Could you check a few things on this model? Use its own coordinates, in mm. Face numbers are marked on the shaded views. A direction names the side the tool comes from. Coordinates: 2 decimals unless noted, no trailing zeros. Order: outer loops, then holes, each group sorted by start corner. A loop starts at its lowest first (then second) coordinate and runs counter-clockwise, first axis right, second up. Notation, with made-up numbers: (44, 77) - (81, 77) arc R20 cw to (81, 112) - close; hole circle Ø11 at (69, 89). An arc over 180 degrees is marked (long way). Answer as CSV lines item,"result". Start each with the question number.
1. I want a section at C-C, the plane z = 17.75. List the corners of the cut face in (x, y) for me.
2. For pin 1 (1.5 mm diameter, centred on y = 19, z = 19, fed in from -X); pin 2 (5 mm diameter, centred on x = -9.5, z = 3.5, fed in from +Y); pin 3 (2.5 mm diameter, centred on y = 18.5, z = 11, fed in from +X), each with a flat end and sliding along its axis, tell me the tip position at first contact or that it passes through.
3. I want a section at B-B, the plane y = 13.25. List the corners of the cut face in (x, z) for me.
4. Thinking about a two-plate mould opening in X: for the marked faces 4, 5 and 6, which applies, released by +X, released by -X, zero draft, split by the parting line, or undercut?
5. For the marked faces 1, 2 and 3, which set-ups out of +Z, -Z, +X, -X, +Y, -Y let a thin tool reach every point of the face, with its end or its side?
6. I want a section at D-D, the plane x = 12.5. List the corners of the cut face in (y, z) for me.
7. I want a section at A-A, the plane x = 24.5. List the corners of the cut face in (y, z) for me.
8. I need wall thicknesses on probe 1 along X at (y, z) = (3.1, 11); probe 2 along X at (y, z) = (22.55, 9); probe 3 along Z at (x, y) = (8, 22). Which ranges of each line are inside material? Lowest first, please.
Autodesk Fusion 360 part; units mm, degrees
sketch "Skizze1" plane through (0, 0, 0) normal (0, 0, 1) x (1, 0, 0)
  line L0 (0, 24) -> (16, 24)
  line L1 (16, 0) -> (0, 0)
  line L2 (2, 22) -> (14, 22)
  line L3 (0, 24) -> (-1, 24)
  line L4 (-1, 24) -> (-1, 0)
  line L5 (-1, 0) -> (0, 0)
  line L6 (16, 24) -> (17, 24)
  line L7 (17, 24) -> (17, 0)
  line L8 (17, 0) -> (16, 0)
  line L9 (2, 22) -> (1, 22)
  line L10 (1, 22) -> (1, 20)
  line L11 (1, 20) -> (2, 20)
  line L12 (15, 20) -> (15, 22)
  line L13 (15, 22) -> (14, 22)
  line L14 (15, 20) -> (2, 20)
  line L15 (2, 20) -> (2, 0)
  line L16 (14, 20) -> (14, 0)
extrude "Extrusion1" add sketch "Skizze1" along normal blind 2
sketch "Skizze2" plane through (0, 0, 2) normal (0, 0, 1) x (-1, 0, 0)
  line L0 (-17, -24) -> (1, -24)
  line L1 (1, -24) -> (1, 0)
  line L2 (1, 0) -> (-17, 0)
  line L3 (-17, 0) -> (-17, -24)
  line L4 (-2, 0) -> (-2, -20)
  line L5 (-2, -20) -> (-1, -20)
  line L6 (-1, -20) -> (-1, -22)
  line L7 (-1, -22) -> (-15, -22)
  line L8 (-15, -22) -> (-15, -20)
  line L9 (-15, -20) -> (-14, -20)
  line L10 (-14, -20) -> (-14, 0)
  line L11 (-2, -20) -> (-14, -20)
extrude "Extrusion2" add sketch "Skizze2" along normal blind 1 contours L0 L1 L2 L3 L4 L5 L6 L7 L8 L9 L10 | L2 L4 L10 L11
sketch "Skizze3" plane through (0, 0, 3) normal (0, 0, 1) x (-1, 0, 0)
  line L0 (-15, -20) -> (-1, -20)
  line L1 (-1, -20) -> (-1, -22)
  line L2 (-1, -22) -> (-15, -22)
  line L3 (-15, -22) -> (-15, -20)
  line L4 (-17, 0) -> (-17, -24)
  line L5 (-17, -24) -> (1, -24)
  line L6 (1, -24) -> (1, 0)
  line L7 (1, 0) -> (-17, 0)
  line L8 (-2, -20) -> (-2, 0)
  line L9 (-14, -20) -> (-14, 0)
extrude "Extrusion3" add sketch "Skizze3" along normal blind 19 contours L0 L1 L2 L3 L4 L5 L6 L7 L8 L9
sketch "Skizze4" plane through (0, 0, 22) normal (0, 0, 1) x (-1, 0, 0)
  line L0 (-2, -20) -> (-1, -20)
  line L1 (-1, -20) -> (-1, -22)
  line L2 (-1, -22) -> (-15, -22)
  line L3 (-15, -22) -> (-15, -20)
  line L4 (-15, -20) -> (-14, -20)
  line L5 (-14, -20) -> (-14, 0)
  line L6 (-14, 0) -> (-17, 0)
  line L7 (-17, 0) -> (-17, -24)
  line L8 (-17, -24) -> (1, -24)
  line L9 (1, -24) -> (1, 0)
  line L10 (1, 0) -> (-2, 0)
  line L11 (-2, 0) -> (-2, -20)
  line L12 (-2, -22) -> (-2, -24)
  line L13 (-14, -22) -> (-14, -24)
extrude "Extrusion4" cut sketch "Skizze4" against normal blind 19 contours L2 L8 L12 L13
sketch "Skizze5" plane through (0, 0, 3) normal (0, 0, 1) x (-1, 0, 0)
  line L0 (-14, 0) -> (-14, -20)
  line L1 (-14, -20) -> (-2, -20)
  line L2 (-2, -20) -> (-2, 0)
  line L3 (-2, 0) -> (-14, 0)
sketch "Skizze6" plane through (0, 0, 3) normal (0, 0, 1) x (1, 0, 0)
sketch "Skizze7" plane through (0, 0, 0) normal (0, 0, 1) x (1, 0, 0)
  line L0 (-1, 0) -> (-16, 0)
  line L1 (-16, 0) -> (-16, 5)
  line L2 (-16, 5) -> (-1, 5)
  line L3 (-1, 5) -> (-1, 0)
  line L4 (17, 0) -> (17, 5)
  line L5 (17, 5) -> (32, 5)
  line L6 (32, 5) -> (32, 0)
  line L7 (32, 0) -> (17, 0)
extrude "Extrusion5" add sketch "Skizze7" along normal blind 22
hole "Bohrung1" at (24.5, 5, 11) direction (0, -1, 0) diameter 2.5 depth 5 tip angle 180 countersink diameter 4.5 countersink angle 90
hole "Bohrung2" at (-8.5, 5, 11) direction (0, -1, 0) diameter 2.5 depth 5 tip angle 180 countersink diameter 4.5 countersink angle 90
extrude "Extrusion6" cut 1 faces at (14.6667, 20, 9) along direction (0, -1, 0) blind 1
extrude "Extrusion7" add 1 faces at (1.3333, 22, 9) along direction (0, -1, 0) blind 1
sketch "Skizze8" plane through (0, 0, 3) normal (0, 0, 1) x (-1, 0, 0)
  line L0 (-14, -21) -> (-14, -24)
  line L1 (-14, -24) -> (-2, -24)
  line L2 (-2, -24) -> (-2, -21)
  line L3 (-2, -21) -> (-14, -21)
  line L4 (-2, -23) -> (-14, -23)
  line L5 (-14, -23) -> (-14, -24)
  line L6 (-14, -24) -> (-2, -24)
  line L7 (-2, -24) -> (-2, -23)
  line L8 (-2, -23) -> (-14, -23)
  line L9 (-14, -23) -> (-14, -24)
extrude "Extrusion8" add sketch "Skizze8" along normal blind 19 contours L0 L1 L2 L4 L5 L6 L7 L8 L9
sketch "Skizze9" plane through (0, 24, 0) normal (0, 1, 0) x (-1, 0, 0)
  line L0 (1, 22) -> (-17, 22)
  line L1 (-17, 22) -> (-17, 0)
  line L2 (-17, 0) -> (1, 0)
  line L3 (1, 0) -> (1, 22)
  line L4 (-8, 0) -> (-8, 9)
hole "Bohrung3" at (8, 24, 9) direction (0, -1, 0) diameter 8 depth 9 tip angle 180
extrude "Extrusion9" cut 1 faces at (14.6667, 19, 9) along direction (0, -1, 0) blind 1.5
extrude "Extrusion10" add 1 faces at (1.3333, 21, 9) along direction (0, -1, 0) blind 1.4
extrude "Extrusion11" add 1 faces at (8, 23, 19) along direction (0, -1, 0) blind 1.2
extrude "Extrusion12" cut 1 faces at (8, 24, 19) along direction (0, -1, 0) blind 1.2
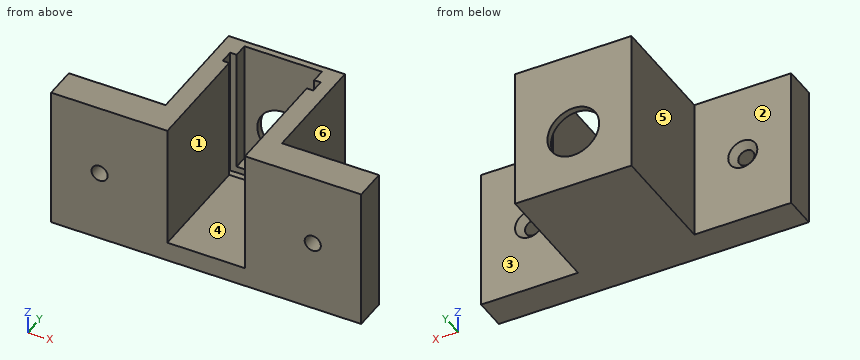
Solved:
1,outline,"(-16, 0) - (2, 0) - (2, 17.5) - (1, 17.5) - (1, 19.6) - (2, 19.6) - (2, 21.8) - (14, 21.8) - (14, 19.6) - (15, 19.6) - (15, 17.5) - (14, 17.5) - (14, 0) - (32, 0) - (32, 5) - (17, 5) - (17, 22.8) - (-1, 22.8) - (-1, 5) - (-16, 5) - close"
2,pin 1,"stops at x = -1"
2,pin 2,"stops at y = 5"
2,pin 3,"stops at x = 17"
3,outline,"(-1, 0) - (17, 0) - (17, 22) - (14, 22) - (14, 3) - (2, 3) - (2, 22) - (-1, 22) - close"
4,face 4,"undercut"
4,face 5,"released by -X"
4,face 6,"released by +X"
5,face 1,"+Z, -Y"
5,face 2,"+Z, -Z, -X, +Y"
5,face 3,"+Z, -Z, +X, +Y"
6,outline,"(0, 0) - (22.8, 0) - (22.8, 22) - (21.8, 22) - (21.8, 3) - (19.6, 3) - (19.6, 2) - (17.5, 2) - (17.5, 3) - (0, 3) - close"
7,outline,"(0, 0) - (5, 0) - (5, 8.75) - (4, 9.75) - (0, 9.75) - close; (0, 12.25) - (4, 12.25) - (5, 13.25) - (5, 22) - (0, 22) - close"
8,probe 1,"x = -16 to -9.75, -7.25 to 2, 14 to 23.25, 25.75 to 32"
8,probe 2,"x = -1 to 4, 12 to 17"
8,probe 3,"z = 0 to 5, 13 to 22"
